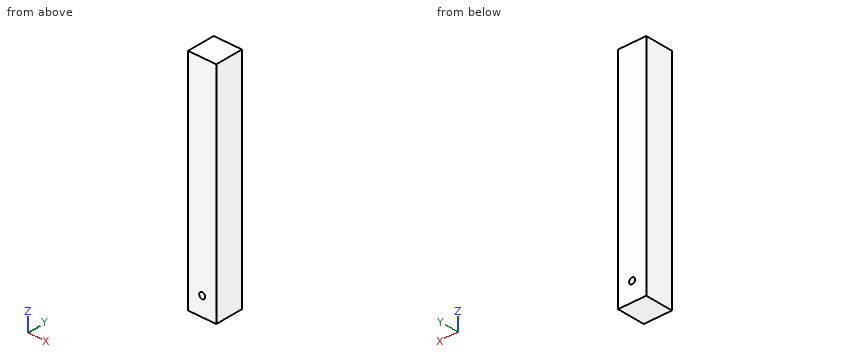
Autodesk Inventor part; units mm, degrees
ref_plane "YZ Plane" through (0, 0, 0) normal (1, 0, 0) x (0, 1, 0)
ref_plane "XZ Plane" through (0, 0, 0) normal (0, 1, 0) x (-1, 0, 0)
ref_plane "XY Plane" through (0, 0, 0) normal (0, 0, 1) x (1, 0, 0)
sketch "スケッチ1" plane through (0, 0, 0) normal (0, 0, 1) x (1, 0, 0)
  line L0 (0, 0) -> (15, 0)
  line L1 (15, 0) -> (15, 15)
  line L2 (15, 15) -> (0, 15)
  line L3 (0, 15) -> (0, 0)
  dimension "d0" = 15
  dimension "d1" = 15
extrude "押し出し1" add sketch "スケッチ1" along normal blind 120
sketch "スケッチ2" plane through (0, 15, 0) normal (0, 1, 0) x (1, 0, 0)
  line L0 (15, 0) -> (0, 0)
  line L1 (15, 0) -> (15, -120)
  point P0 (7.5, -10)
  dimension "d4" = 10
  dimension "d5" = 7.5
hole "穴1" at (7.5, 15, 10) direction (0, -1, 0) diameter 3.2 end through all
properties part number "射出_角柱7"
The listing builds one solid part. Answer for the finished solid, in the listing's coordinates (mm). Give positions to 0.01 mm unless a question says otherwise; leave off trailing zeros. Write each loop counter-clockwise with the first axis right and the second up, starting at its lowest first coordinate (ties: lowest second). Pieces come first, ordered by that corner, then holes.
Item 1: Find the intervals of material crossed by line 1 along X through (y, z) = (9.75, 10); line 2 along Z through (x, y) = (7.5, 8.5); line 3 along Z through (x, y) = (6.5, 13), in increasing order.
Item 2: Section B-B, the plane x = 7.5 is taken. Write down the section's boundary in (y, z).
Item 3: Section A-A, the plane z = 10 is taken. Write down the section's boundary in (x, y), plus the area to 3 significant figures.
Completed:
1. line 1: x = 0 to 5.9, 9.1 to 15
1. line 2: z = 0 to 8.4, 11.6 to 120
1. line 3: z = 0 to 8.75, 11.25 to 120
2. outline: (0, 0) - (15, 0) - (15, 8.4) - (0, 8.4) - close; (0, 11.6) - (15, 11.6) - (15, 120) - (0, 120) - close
3. outline: (0, 0) - (5.9, 0) - (5.9, 15) - (0, 15) - close; (9.1, 0) - (15, 0) - (15, 15) - (9.1, 15) - close
3. area: 177 mm2
